Work out the finished part from the listing and answer in its coordinate system (mm). Face numbers are marked on the shaded views. Coordinates: 2 decimals unless noted, no trailing zeros. Loops run counter-clockwise (first coordinate to the right, second up) from the corner with the lowest first, then second, coordinate; pieces in that order, holes last. Notation, with made-up numbers: (4.5, 30) - (10.5, 30) arc R21 ccw to (10.5, 46) - close; hole circle Ø3 at (64.5, -32.5). An arc over 180 degrees is marked (long way). Write each question's results on one line, items separated by ' | '. Start each with the question number.
1. A cutting plane is placed at A-A on y = 0. Determine the outline of the cut face in (x, z), then the cut area to 3 significant figures.
2. Find the intervals of material crossed by line 1 along Z through (x, y) = (-3.5, -11.5); line 2 along X through (y, z) = (0.5, 2.5); line 3 along Y through (x, z) = (16, 14.5), in increasing order. Write a range as [from, to].
3. A cutting plane is placed at D-D on x = 14. Determine the outline of the cut face in (y, z), then the cut area to 3 significant figures.
4. Each of these flat-tipped pins is pushed along its axis until it touches: P1, Ø10, axis at x = -12, z = 28, coming from the -Y side; P2, Ø3, axis at x = 7.5, z = 70.5, coming from the +Y side; P3, Ø13.5, axis at x = -0.5, y = -8.5, coming from the +Z side; P4, Ø8, axis at x = 9.5, y = 17.5, coming from the -Z side. Where does it stop, or does it pass through?
5. A cutting plane is placed at C-C on y = -11.5. Determine the outline of the cut face in (x, z).
6. Determine the mould class of the marked faces 1, 2 and 3 for opening direction Z: released by +Z, released by -Z, zero draft, split by the parting line, or undercut.
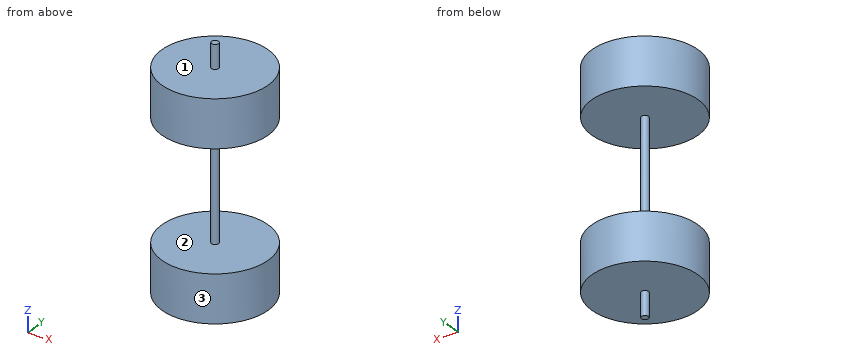
from build123d import *

# Parameters (mm, degrees)
ESBO_O1_R                = 22.5
RESSALTO_EXTRUS_O3_DEPTH = 20
ESBO_O3_R                = 1.5
RESSALTO_EXTRUS_O4_DEPTH = 50
ESBO_O4_R                = 22.5
RESSALTO_EXTRUS_O5_DEPTH = 20
ESBO_O5_R                = 1.5
RESSALTO_EXTRUS_O6_DEPTH = 10
RESSALTO_EXTRUS_O7_START = 10
ESBO_O6_R                = 1.5
RESSALTO_EXTRUS_O7_DEPTH = 10


with BuildPart() as part:
    # Esboço1 → Ressalto-extrusão3 (new body)
    with BuildSketch(Plane.XY):
        Circle(ESBO_O1_R)
    extrude(amount=RESSALTO_EXTRUS_O3_DEPTH)

    # Esboço3 → Ressalto-extrusão4 (add)
    with BuildSketch(Plane.XY.offset(20)):
        Circle(ESBO_O3_R)
    extrude(amount=RESSALTO_EXTRUS_O4_DEPTH)

    # Esboço4 → Ressalto-extrusão5 (add)
    with BuildSketch(Plane.XY.offset(70)):
        Circle(ESBO_O4_R)
    extrude(amount=RESSALTO_EXTRUS_O5_DEPTH)

    # Esboço5 → Ressalto-extrusão6 (add)
    with BuildSketch(Plane.XY.offset(90)):
        Circle(ESBO_O5_R)
    extrude(amount=RESSALTO_EXTRUS_O6_DEPTH)

    # Esboço6 → Ressalto-extrusão7 (add)
    with BuildSketch(Plane(origin=(0, 0, 0), x_dir=(-1, 0, 0), z_dir=(0, 0, -1)).offset(RESSALTO_EXTRUS_O7_START)):
        with Locations(Location((0, 0, 0), (0, 0, 180))):
            Circle(ESBO_O6_R)
    extrude(amount=-RESSALTO_EXTRUS_O7_DEPTH)


solid = part.part
Values:
1) outline: (-22.5, 0) - (-1.5, 0) - (-1.5, -10) - (1.5, -10) - (1.5, 0) - (22.5, 0) - (22.5, 20) - (1.5, 20) - (1.5, 70) - (22.5, 70) - (22.5, 90) - (1.5, 90) - (1.5, 100) - (-1.5, 100) - (-1.5, 90) - (-22.5, 90) - (-22.5, 70) - (-1.5, 70) - (-1.5, 20) - (-22.5, 20) - close | area: 2,010 mm^2
2) line 1: [0, 20], [70, 90] | line 2: [-22.49, 22.49] | line 3: [-15.82, 15.82]
3) outline: (-17.61, 0) - (17.61, 0) - (17.61, 20) - (-17.61, 20) - close; (-17.61, 70) - (17.61, 70) - (17.61, 90) - (-17.61, 90) - close | area: 1,410 mm^2
4) P1: through | P2: y = 21.69 | P3: z = 90 | P4: z = 0
5) outline: (-19.34, 0) - (19.34, 0) - (19.34, 20) - (-19.34, 20) - close; (-19.34, 70) - (19.34, 70) - (19.34, 90) - (-19.34, 90) - close
6) face 1: released by +Z | face 2: undercut | face 3: zero draft
